Source: CAD feature listing. Evaluate the final solid. Frame: model axes, mm. A direction names the side the tool comes from. Give positions to 0.01 mm unless a question says otherwise; leave off trailing zeros. Order: outer loops, then holes, each group sorted by start corner. A loop starts at its lowest first (then second) coordinate and runs counter-clockwise, first axis right, second up.
1) First-contact query: P1, Ø3, axis at x = 1, z = 8.5, coming from the -Y side; P2, Ø15, axis at x = 1, y = -12.5, coming from the +Z side; P3, Ø3, axis at y = -24.5, z = 7, coming from the -X side; P4, Ø5, axis at x = 30, y = 92.5, coming from the -Z side. Flat tips, straight axial feed; report the tip coordinate or a pass-through.
2) Draft query along X for faces 3 (the face through (40, 48, 8)), 4 (the face through (1, 100, 8)), 5 (the face through (2.9, 23, 10)). Return one class per face: released by +X, released by -X, zero draft, split by the parting line, or undercut.
3) Section A-A, the plane y = 92.5. Return loops of the section in (x, z).
4) Section B-B, the plane z = 12.25. Return loops of the section in (x, y).
5) Material intervals for line 1 (Y direction, x = 0, z = 11.5); line 2 (X direction, y = 0, z = 7.25); line 3 (Y direction, x = -1, z = 7.75), sorted ascending.
6) Access query for faces 1 (the face through (0, 21.132, 10)), 2 (the face through (-1, 47, 15)). Directions: +Z, -Z, +X, -X, +Y, -Y. A direction counts if a zero-diameter tool reaches every point of the face in a straight line with its end or side. Return the directions, or none.
7) Section C-C, the plane x = 0. Return loops of the section in (y, z), plus the area to 3 significant figures.
```python
from build123d import *

# Parameters (mm, degrees)
SKETCH1_R           = 40
BOSS_EXTRUDE1_DEPTH = 15
SKETCH2_R           = 25.1
CUT_EXTRUDE1_DEPTH  = 10
BOSS_EXTRUDE2_DEPTH = 10
CHAMFER1_SIZE       = 1
BOSS_EXTRUDE3_DEPTH = 15
SKETCH5_R           = 2.25
CUT_EXTRUDE2_DEPTH  = 109.742815855
FILLET1_R           = 2


with BuildPart() as part:
    # Sketch1 → Boss-Extrude1 (new body)
    with BuildSketch(Plane.XY):
        Circle(SKETCH1_R)
    extrude(amount=BOSS_EXTRUDE1_DEPTH)

    # Sketch2 → Cut-Extrude1 (cut)
    with BuildSketch(Plane.XY.offset(15)):
        Circle(SKETCH2_R)
    extrude(amount=-CUT_EXTRUDE1_DEPTH, mode=Mode.SUBTRACT)

    # Sketch3 → Boss-Extrude2 (add)
    with BuildSketch(Plane.XY.offset(15)):
        with BuildLine():
            Line((2.9, 21.131907268), (-2.9, 21.131907268))
            Line((-2.9, 21.131907268), (-2.9, 24.931907268))
            ThreePointArc((-2.9, 24.931907268), (0, 25.1), (2.9, 24.931907268))
            Line((2.9, 24.931907268), (2.9, 21.131907268))
        make_face()
    extrude(amount=-BOSS_EXTRUDE2_DEPTH)

    # Chamfer1
    chamfer1_edges = [part.edges().sort_by_distance(p)[0] for p in [
        (0, -25.1, 15),
        (-2.9, 23.031907268, 15),
        (0, 21.131907268, 15),
        (2.9, 23.031907268, 15),
    ]]
    chamfer(chamfer1_edges, length=CHAMFER1_SIZE)

    # Sketch4 → Boss-Extrude3 (add, through all)
    with BuildSketch(Plane(origin=(0, 0, 0), x_dir=(-1, 0, 0), z_dir=(0, 0, -1))):
        with BuildLine():
            Line((-40, 0), (-40, 100))
            Line((-40, 100), (40, 100))
            Line((40, 100), (40, 0))
            ThreePointArc((40, 0), (0, 40), (-40, 0))
        make_face()
    extrude(amount=-BOSS_EXTRUDE3_DEPTH)

    # Sketch5 → Cut-Extrude2 (cut, through all)
    with BuildSketch(Plane(origin=(0, 0, 0), x_dir=(-1, 0, 0), z_dir=(0, 0, -1))):
        with Locations((0, 92.5)):
            Circle(SKETCH5_R)
        with Locations((-30, 92.5)):
            Circle(SKETCH5_R)
        with Locations(Location((30, 92.5, 0), (0, 0, 180))):
            Circle(SKETCH5_R)
    extrude(amount=-CUT_EXTRUDE2_DEPTH, mode=Mode.SUBTRACT)

    # Fillet1
    fillet1_edges = [part.edges().sort_by_distance(p)[0] for p in [
        (0, -40, 0),
        (40, 100, 7.5),
        (-40, 100, 7.5),
        (-40, 50, 0),
        (0, 100, 0),
        (40, 50, 0),
    ]]
    fillet(fillet1_edges, radius=FILLET1_R)


solid = part.part
```
From the geometry:
1. P1: stops at y = -40
1. P2: stops at z = 5
1. P3: stops at x = -32.73
1. P4: stops at z = 0
2. face 3: released by +X
2. face 4: zero draft
2. face 5: undercut
3. outline: (-40, 2) arc R2 ccw to (-38, 0) - (-32.25, 0) - (-32.25, 15) - (-40, 15) - close; (-27.75, 0) - (-2.25, 0) - (-2.25, 15) - (-27.75, 15) - close; (2.25, 0) - (27.75, 0) - (27.75, 15) - (2.25, 15) - close; (32.25, 0) - (38, 0) arc R2 ccw to (40, 2) - (40, 15) - (32.25, 15) - close
4. outline: (-40, 0) arc R40 ccw to (40, 0) - (40, 98) arc R2 ccw to (38, 100) - (-38, 100) arc R2 ccw to (-40, 98) - close; hole circle Ø4.5 at (-30, 92.5); hole (-2.9, 21.13) - (-2.9, 24.93) arc R25.1 ccw (long way) to (2.9, 24.93) - (2.9, 21.13) - close; hole circle Ø4.5 at (0, 92.5); hole circle Ø4.5 at (30, 92.5)
5. line 1: y = -40 to -25.1, 21.13 to 90.25, 94.75 to 100
5. line 2: x = -40 to -25.1, 25.1 to 40
5. line 3: y = -39.99 to -25.08, 21.13 to 90.48, 94.52 to 100
6. face 1: +Z
6. face 2: +Z, +X, -X, +Y, -Y
7. outline: (-40, 2) arc R2 ccw to (-38, 0) - (90.25, 0) - (90.25, 15) - (22.13, 15) - (21.13, 14) - (21.13, 5) - (-25.1, 5) - (-25.1, 14) - (-26.1, 15) - (-40, 15) - close; (94.75, 0) - (98, 0) arc R2 ccw to (100, 2) - (100, 15) - (94.75, 15) - close
7. area: 1,570 mm2
